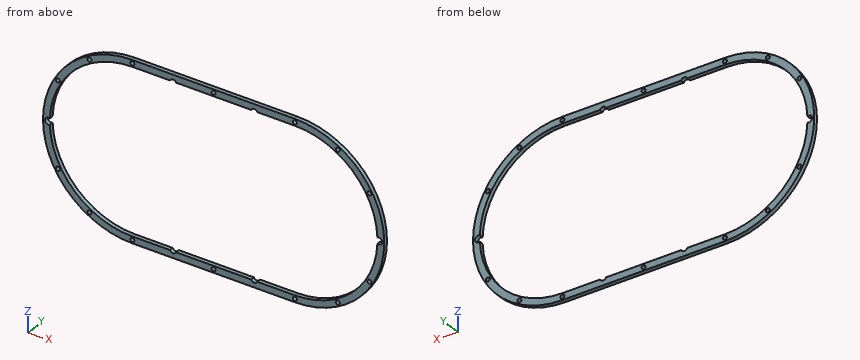
```python
from build123d import *

# Parameters (mm, degrees)
SKETCH_1_R          = 1.5
EXTRUDE_2_DEPTH     = 3
CUT_EXTRUDE_1_DEPTH = 10
SKETCH_4_R          = 7.5
CUT_EXTRUDE_2_DEPTH = 10
SKETCH_5_R          = 1.5
CUT_EXTRUDE_3_DEPTH = 10
CUT_EXTRUDE_4_DEPTH = 10


with BuildPart() as part:
    # 草图1 → 凸台-拉伸2 (new body)
    with BuildSketch(Plane(origin=(0, 0, 0), x_dir=(1, 0, 0), z_dir=(0, 1, 0))):
        with BuildLine():
            Line((-60, 70), (60, 70))
            ThreePointArc((60, 70), (130, 0), (60, -70))
            Line((60, -70), (-60, -70))
            ThreePointArc((-60, -70), (-130, 0), (-60, 70))
        make_face()
        with Locations((-122, 0)):
            Circle(SKETCH_1_R, mode=Mode.SUBTRACT)
        with Locations((122, 0)):
            Circle(SKETCH_1_R, mode=Mode.SUBTRACT)
        with Locations((-30, 60)):
            Circle(SKETCH_1_R, mode=Mode.SUBTRACT)
        with Locations((30, 60)):
            Circle(SKETCH_1_R, mode=Mode.SUBTRACT)
        with Locations((30, -60)):
            Circle(SKETCH_1_R, mode=Mode.SUBTRACT)
        with Locations((-30, -60)):
            Circle(SKETCH_1_R, mode=Mode.SUBTRACT)
    extrude(amount=EXTRUDE_2_DEPTH)

    # 草图3 → 切除-拉伸1 (cut)
    with BuildSketch(Plane(origin=(0, 3, 0), x_dir=(1, 0, 0), z_dir=(0, 1, 0))):
        with BuildLine():
            Line((-60, -70), (60, -70))
            ThreePointArc((60, -70), (130, 0), (60, 70))
            Line((60, 70), (-60, 70))
            ThreePointArc((-60, 70), (-130, 0), (-60, -70))
        make_face()
        with BuildLine():
            Line((-60, -66), (60, -66))
            ThreePointArc((60, -66), (126, 0), (60, 66))
            Line((60, 66), (-60, 66))
            ThreePointArc((-60, 66), (-126, 0), (-60, -66))
        make_face(mode=Mode.SUBTRACT)
    extrude(amount=-CUT_EXTRUDE_1_DEPTH, mode=Mode.SUBTRACT)

    # 草图4 → 切除-拉伸2 (cut)
    with BuildSketch(Plane(origin=(0, 3, 0), x_dir=(1, 0, 0), z_dir=(0, 1, 0))):
        with Locations((-96, 0)):
            Circle(SKETCH_4_R)
        with Locations((96, 0)):
            Circle(SKETCH_4_R)
        with Locations((0, 36)):
            Circle(SKETCH_4_R)
        with Locations((0, -36)):
            Circle(SKETCH_4_R)
        with Locations((-60, -36)):
            Circle(SKETCH_4_R)
        with Locations((60, -36)):
            Circle(SKETCH_4_R)
        with Locations((30, -36)):
            Circle(SKETCH_4_R)
        with Locations((-30, -36)):
            Circle(SKETCH_4_R)
        with Locations((-85.455844123, -25.455844123)):
            Circle(SKETCH_4_R)
        with Locations((60, 36)):
            Circle(SKETCH_4_R)
        with Locations((30, 36)):
            Circle(SKETCH_4_R)
        with Locations((-85.455844123, 25.455844123)):
            Circle(SKETCH_4_R)
        with Locations((-30, 36)):
            Circle(SKETCH_4_R)
        with Locations((-60, 36)):
            Circle(SKETCH_4_R)
        with Locations((85.455844123, -25.455844123)):
            Circle(SKETCH_4_R)
        with Locations((85.455844123, 25.455844123)):
            Circle(SKETCH_4_R)
    extrude(amount=-CUT_EXTRUDE_2_DEPTH, mode=Mode.SUBTRACT)

    # 草图5 → 切除-拉伸3 (cut)
    with BuildSketch(Plane(origin=(0, 3, 0), x_dir=(1, 0, 0), z_dir=(0, 1, 0))):
        with Locations((-60, 63.5)):
            Circle(SKETCH_5_R)
        with Locations((114.99261314, 31.75)):
            Circle(SKETCH_5_R)
        with Locations((0, 63.5)):
            Circle(SKETCH_5_R)
        with Locations((60, 63.5)):
            Circle(SKETCH_5_R)
        with Locations((91.75, 54.99261314)):
            Circle(SKETCH_5_R)
        with Locations((91.75, -54.99261314)):
            Circle(SKETCH_5_R)
        with Locations((114.99261314, -31.75)):
            Circle(SKETCH_5_R)
        with Locations((-91.75, -54.99261314)):
            Circle(SKETCH_5_R)
        with Locations((-114.99261314, -31.75)):
            Circle(SKETCH_5_R)
        with Locations((-91.75, 54.99261314)):
            Circle(SKETCH_5_R)
        with Locations((-114.99261314, 31.75)):
            Circle(SKETCH_5_R)
        with Locations((60, -63.5)):
            Circle(SKETCH_5_R)
        with Locations((0, -63.5)):
            Circle(SKETCH_5_R)
        with Locations((-60, -63.5)):
            Circle(SKETCH_5_R)
    extrude(amount=-CUT_EXTRUDE_3_DEPTH, mode=Mode.SUBTRACT)

    # 草图6 → 切除-拉伸4 (cut)
    with BuildSketch(Plane(origin=(0, 3, 0), x_dir=(1, 0, 0), z_dir=(0, 1, 0))):
        with BuildLine():
            Line((60, 61), (32.291287847, 61))
            ThreePointArc((32.291287847, 61), (30, 62.5), (27.708712153, 61))
            Line((27.708712153, 61), (-27.708712153, 61))
            ThreePointArc((-27.708712153, 61), (-30, 62.5), (-32.291287847, 61))
            Line((-32.291287847, 61), (-60, 61))
            ThreePointArc((-60, 61), (-102.322495481, 43.929561531), (-120.95766129, 2.272340207))
            ThreePointArc((-120.95766129, 2.272340207), (-124.5, 0), (-120.95766129, -2.272340207))
            ThreePointArc((-120.95766129, -2.272340207), (-102.322495481, -43.929561531), (-60, -61))
            Line((-60, -61), (-32.291287847, -61))
            ThreePointArc((-32.291287847, -61), (-30, -62.5), (-27.708712153, -61))
            Line((-27.708712153, -61), (27.708712153, -61))
            ThreePointArc((27.708712153, -61), (30, -62.5), (32.291287847, -61))
            Line((32.291287847, -61), (60, -61))
            ThreePointArc((60, -61), (102.322495481, -43.929561531), (120.95766129, -2.272340207))
            ThreePointArc((120.95766129, -2.272340207), (124.5, 0), (120.95766129, 2.272340207))
            ThreePointArc((120.95766129, 2.272340207), (102.322495481, 43.929561531), (60, 61))
        make_face()
    extrude(amount=-CUT_EXTRUDE_4_DEPTH, mode=Mode.SUBTRACT)


solid = part.part
```
Source: CAD feature listing. Evaluate the final solid. Frame: model axes, mm. Give positions to 0.01 mm unless a question says otherwise; leave off trailing zeros. Write each loop counter-clockwise with the first axis right and the second up, starting at its lowest first coordinate (ties: lowest second). Pieces come first, ordered by that corner, then holes. Notation, with made-up numbers: (42, 34) - (101, 34) arc R22 ccw to (101, 61) - close; hole circle Ø9 at (10.5, 65.25). An arc over 180 degrees is marked (long way). One line per item, written item: value. Start each with the question number.
Q1. Section query B-B, the plane z = -12. Return the cut outline in (x, y), then the cut area to 3 significant figures.
Q2. Material intervals for probe 1 along Z at (x, y) = (-60, 1.9); probe 2 along Z at (x, y) = (52.5, 1.2); probe 3 along Z at (x, y) = (-91.75, 1), sorted ascending. Write a range as from..to.
Q3. First-contact query: pin 1 Ø3.5 at (x, z) = (0, -63.5) entering from +Y; pin 2 Ø1.8 at (x, z) = (-60, 63.5) entering from +Y; pin 3 Ø1.5 at (y, z) = (1.5, 22) entering from +X. Flat tips, straight axial feed; report the tip coordinate or a pass-through.
Q4. Section query A-A, the plane x = -69. Return the cut outline in (y, z).
Q5. Section query C-C, the plane y = 1.8. Count the separate pieces of the cut face and the enclosed holes in it, then the cut area to 3 significant figures.
Answer:
1. outline: (-124.9, 0) - (-119.81, 0) - (-119.81, 3) - (-124.9, 3) - close; (119.81, 0) - (124.9, 0) - (124.9, 3) - (119.81, 3) - close
1. area: 30.6 mm2
2. probe 1: z = -66..-65, -62..-61, 61..62, 65..66
2. probe 2: z = -66..-61, 61..66
2. probe 3: z = -57.86..-56.49, -53.49..-52.09, 52.09..53.49, 56.49..57.86
3. pin 1: stops at y = 3
3. pin 2: passes through
3. pin 3: stops at x = 122.49
4. outline: (0, -65.38) - (3, -65.38) - (3, -60.33) - (0, -60.33) - close; (0, 60.33) - (3, 60.33) - (3, 65.38) - (0, 65.38) - close
5. separate pieces: 1
5. enclosed holes: 15
5. area: 3,050 mm2
